from build123d import *

# Parameters (mm, degrees)
SKICA1_R                = 2.125
SKICA1_W                = 20
SKICA1_H                = 4
SKICA1_H_2              = 35
SKICA1_R_2              = 2
SKICA1_W_2              = 80
SKICA1_H_3              = 60
SKICA1_R_3              = 60
SKICA1_R_4              = 1.5
SKICA1_W_3              = 15
SKICA1_H_4              = 20
P_IDAT_VYSUNUT_M1_DEPTH = 4


with BuildPart() as part:
    # Skica1 → Přidat vysunutím1 (new body)
    with BuildSketch(Plane.XY):
        Polygon((0, 0), (0, 10), (4, 10), (4, 30), (0, 30), (0, 50), (4, 50), (4, 70), (0, 70), (0, 90), (4, 90), (4, 110), (0, 110), (0, 130), (4, 130), (4, 150), (0, 150), (0, 170), (4, 170), (4, 190), (0, 190), (0, 210), (-44.218272824, 270), (-77.5, 270), (-77.5, 317), (-122.5, 317), (-122.5, 270), (-155.781727176, 270), (-200, 210), (-200, 190), (-204, 190), (-204, 170), (-200, 170), (-200, 150), (-204, 150), (-204, 130), (-200, 130), (-200, 110), (-204, 110), (-204, 90), (-200, 90), (-200, 70), (-204, 70), (-204, 50), (-200, 50), (-200, 30), (-204, 30), (-204, 10), (-200, 10), (-200, 0), (-190, 0), (-190, -4), (-170, -4), (-170, 0), (-150, 0), (-150, -4), (-130, -4), (-130, 0), (-70, 0), (-70, -4), (-50, -4), (-50, 0), (-30, 0), (-30, -4), (-10, -4), (-10, 0), align=None)
        with Locations((-185.5, 3.5)):
            Circle(SKICA1_R, mode=Mode.SUBTRACT)
        with Locations((-185.5, 28)):
            Circle(SKICA1_R, mode=Mode.SUBTRACT)
        with Locations((-180, 82)):
            Rectangle(SKICA1_W, SKICA1_H, mode=Mode.SUBTRACT)
        with Locations((-180, 124)):
            Rectangle(SKICA1_W, SKICA1_H, mode=Mode.SUBTRACT)
        with Locations((-182.785843761, 152.5)):
            Rectangle(SKICA1_W, SKICA1_H_2, mode=Mode.SUBTRACT)
        with Locations((-155.781727176, 147.5)):
            Circle(SKICA1_R_2, mode=Mode.SUBTRACT)
        with Locations((-140, 124)):
            Rectangle(SKICA1_W, SKICA1_H, mode=Mode.SUBTRACT)
        with Locations((-14.5, 3.5)):
            Circle(SKICA1_R, mode=Mode.SUBTRACT)
        with Locations((-14.5, 28)):
            Circle(SKICA1_R, mode=Mode.SUBTRACT)
        with Locations((-100, 80)):
            Rectangle(SKICA1_W_2, SKICA1_H_3, mode=Mode.SUBTRACT)
        with Locations((-60, 124)):
            Rectangle(SKICA1_W, SKICA1_H, mode=Mode.SUBTRACT)
        with Locations((-50.781727176, 147.5)):
            Circle(SKICA1_R_2, mode=Mode.SUBTRACT)
        with Locations((-20, 82)):
            Rectangle(SKICA1_W, SKICA1_H, mode=Mode.SUBTRACT)
        with Locations((-20, 124)):
            Rectangle(SKICA1_W, SKICA1_H, mode=Mode.SUBTRACT)
        with Locations((-17.214156239, 152.5)):
            Rectangle(SKICA1_W, SKICA1_H_2, mode=Mode.SUBTRACT)
        with Locations((-103.281727176, 200)):
            Circle(SKICA1_R_3, mode=Mode.SUBTRACT)
        with Locations((-155.781727176, 252.5)):
            Circle(SKICA1_R_2, mode=Mode.SUBTRACT)
        with Locations((-50.781727176, 252.5)):
            Circle(SKICA1_R_2, mode=Mode.SUBTRACT)
        with Locations((-89.5, 301)):
            Circle(SKICA1_R_4, mode=Mode.SUBTRACT)
        with Locations((-110.5, 288.5)):
            Circle(SKICA1_R_4, mode=Mode.SUBTRACT)
        with Locations((-100, 295)):
            Rectangle(SKICA1_W_3, SKICA1_H_4, mode=Mode.SUBTRACT)
        with Locations((-110.5, 301)):
            Circle(SKICA1_R_4, mode=Mode.SUBTRACT)
        with Locations((-89.5, 288.5)):
            Circle(SKICA1_R_4, mode=Mode.SUBTRACT)
    extrude(amount=P_IDAT_VYSUNUT_M1_DEPTH)


solid = part.part
CAD build for the part. Positions are in the model's coordinates, mm. Coordinates: 2 decimals unless noted, no trailing zeros. Order: outer loops, then holes, each group sorted by start corner. A loop starts at its lowest first (then second) coordinate and runs counter-clockwise, first axis right, second up.
Item 1: Band-saw the part on B-B on x = -144. List the corners of the cut face in (y, z).
Check sheet entries:
outline: (-4, 0) - (122, 0) - (122, 4) - (-4, 4) - close; (126, 0) - (155.93, 0) - (155.93, 4) - (126, 4) - close; (244.07, 0) - (270, 0) - (270, 4) - (244.07, 4) - close
Item 2: Band-saw the part on C-C on y = 161.5. List the corners of the cut face in (x, z).
Check sheet entries:
outline: (-200, 0) - (-192.79, 0) - (-192.79, 4) - (-200, 4) - close; (-172.79, 0) - (-149.3, 0) - (-149.3, 4) - (-172.79, 4) - close; (-57.26, 0) - (-27.21, 0) - (-27.21, 4) - (-57.26, 4) - close; (-7.21, 0) - (0, 0) - (0, 4) - (-7.21, 4) - close
Item 3: Band-saw the part on D-D on z = 2.3. Give the number of separate pieces and of enclosed holes in the cut face, plus the area to 3 significant figures.
Check sheet entries:
separate pieces: 1
enclosed holes: 23
area: 36,200 mm2
Item 4: Drill centre lines: L1, parallel to X at y = 122.5, z = 1.7; L2, parallel to Y at x = -65.5, z = 0.5; L3, parallel to Y at x = -121, z = 1.1. Where is each one in solid material? Low to high.
Check sheet entries:
L1: x = -200 to -190, -170 to -150, -130 to -70, -50 to -30, -10 to 0
L2: y = -4 to 50, 110 to 122, 126 to 153.39, 246.61 to 270
L3: y = 0 to 50, 110 to 142.68, 257.32 to 317
Item 5: Two-plate mould, pull along Z, no slides. Class faces 1 (the face through (-101, 123, 0)), 2 (the face through (-101, 123, 4)), 3 (the face through (-177.58, 240.42, 1.97)): +Z half, -Z half, draft (parallel to the pull), parting line (faces both ways), or undercut.
Check sheet entries:
face 1: -Z half
face 2: +Z half
face 3: draft
Item 6: Band-saw the part on A-A on y = 66. List the corners of the cut face in (x, z).
Check sheet entries:
outline: (-204, 0) - (-140, 0) - (-140, 4) - (-204, 4) - close; (-60, 0) - (4, 0) - (4, 4) - (-60, 4) - close
Item 7: Pin check, flat tips, straight feed: pin 1 Ø1.2 at (y, z) = (124, 2) entering from +X; pin 2 Ø1.2 at (x, z) = (2.5, 1) entering from +Y; pin 3 Ø1.2 at (y, z) = (7, 1.5) entering from -X. Stop position of each tip, or through.
Check sheet entries:
pin 1: stops at x = 0
pin 2: stops at y = 190
pin 3: stops at x = -200
